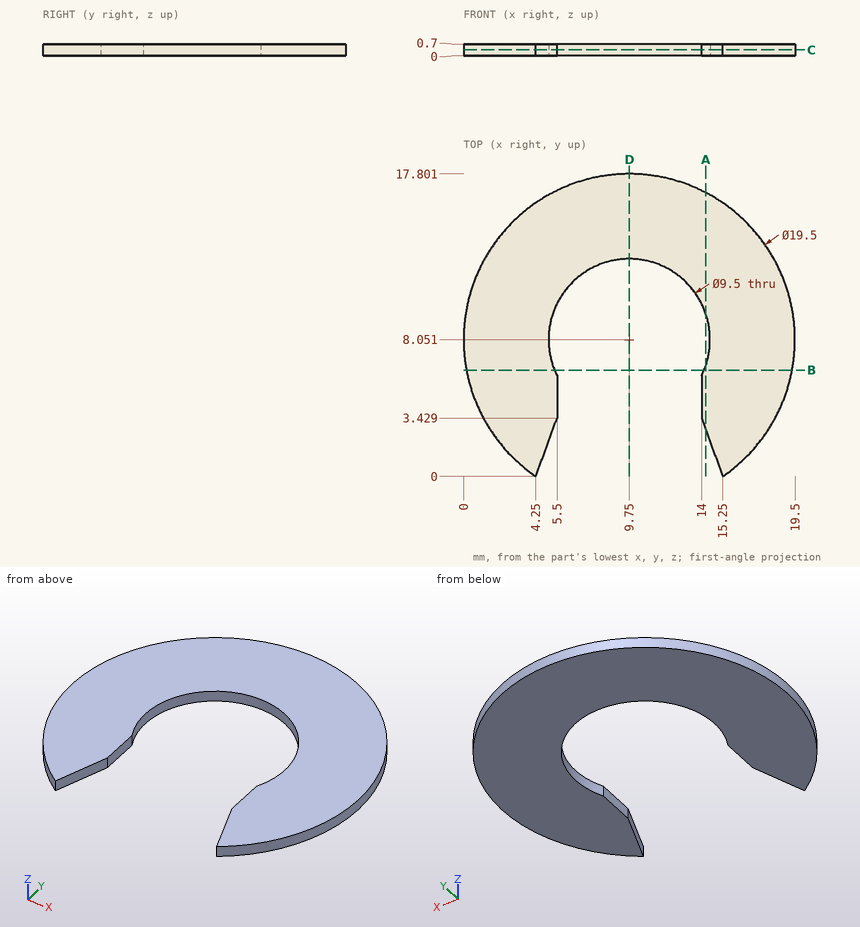
The figure shows three views and two pictorial views of one solid part (mm, origin at its lowest corner). Answer the questions. Round coordinates to 2 decimals unless told otherwise and drop trailing zeros. Order: outer loops, then holes, each group sorted by start corner. A loop starts at its lowest first (then second) coordinate and runs counter-clockwise, first axis right, second up. Notation, with made-up numbers: (1.25, 72) - (32.25, 72) arc R24 cw to (32.25, 97) - close; hole circle Ø4 at (38, -0.75). An arc over 180 degrees is marked (long way). Write item = value, one per line. Start each with the question number.
1) Section A-A, the plane x = 14.25 is taken. Write down the section's boundary in (y, z).
2) Section D-D, the plane x = 9.75 is taken. Write down the section's boundary in (y, z).
3) Section C-C, the plane z = 0.35 is taken. Write down the section's boundary in (x, y).
4) Section B-B, the plane y = 6.25 is taken. Write down the section's boundary in (x, z) (1 decimal).
5) Straight lines are drawn through the part: L1, parallel to Y at x = 9.75, z = 0.2; L2, parallel to X at y = 2, z = 0.2 (1 decimal); L3, parallel to X at y = 6, z = 0.1 (1 decimal). For each, find the intervals that lie inside material, in ascending order.
Results list:
q1.outline = (2.74, 0) - (6.53, 0) - (6.53, 0.7) - (2.74, 0.7) - close; (9.57, 0) - (16.7, 0) - (16.7, 0.7) - (9.57, 0.7) - close
q2.outline = (12.8, 0) - (17.8, 0) - (17.8, 0.7) - (12.8, 0.7) - close
q3.outline = (4.25, 0) - (5.5, 3.43) - (5.5, 5.93) arc R4.75 cw (long way) to (14, 5.93) - (14, 3.43) - (15.25, 0) arc R9.75 ccw (long way) to start
q4.outline = (0.2, 0) - (5.4, 0) - (5.4, 0.7) - (0.2, 0.7) - close; (14.1, 0) - (19.3, 0) - (19.3, 0.7) - (14.1, 0.7) - close
q5.L1 = 12.8 to 17.8
q5.L2 = 2.1 to 5, 14.5 to 17.4
q5.L3 = 0.2 to 5.5, 14 to 19.3
